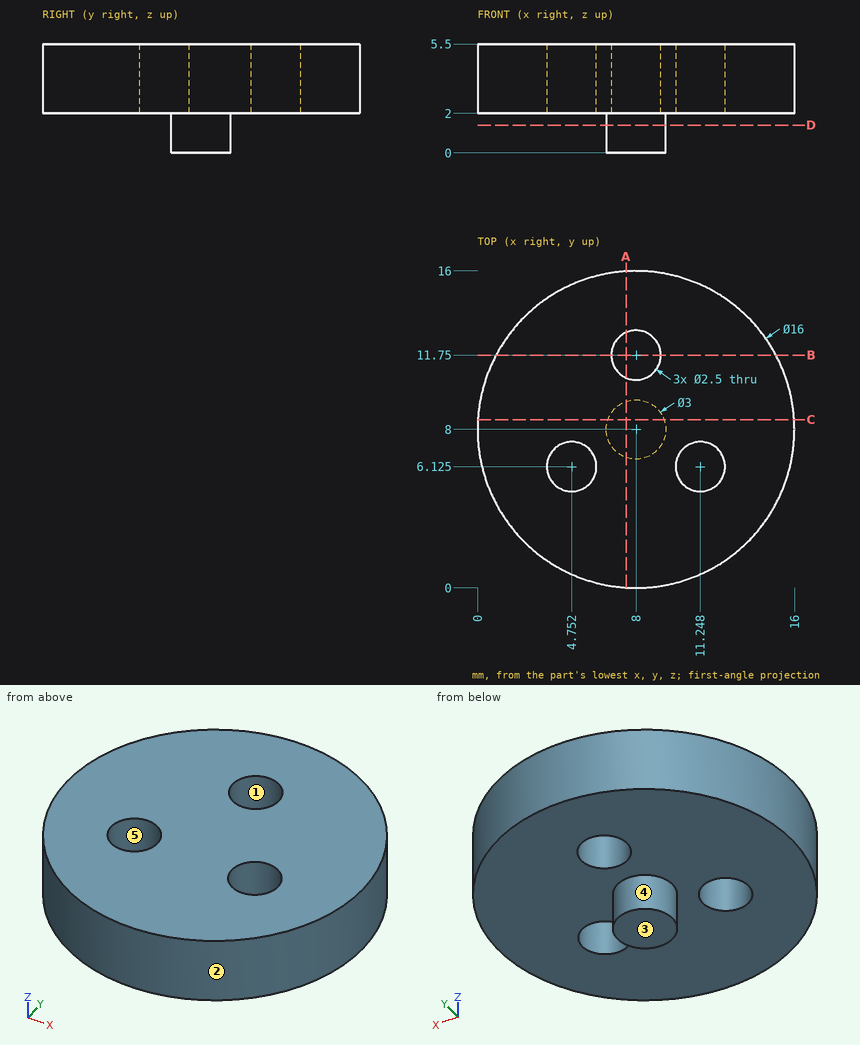
Geometry check sheet. Reference: drawing and pictorial views, mm from the part's lowest x, y, z. A direction names the side the tool comes from. Round coordinates to 2 decimals unless told otherwise and drop trailing zeros. Write each loop counter-clockwise with the first axis right and the second up, starting at its lowest first coordinate (ties: lowest second). Pieces come first, ordered by that corner, then holes.
Item 1: Section check B-B (y = 11.75). Record the boundary of the cut face in (x, z), plus the area to 3 significant figures.
Determined:
outline: (0.93, 2) - (6.75, 2) - (6.75, 5.5) - (0.93, 5.5) - close; (9.25, 2) - (15.07, 2) - (15.07, 5.5) - (9.25, 5.5) - close
area: 40.7 mm2
Item 2: Mould release check, pull along X, two halves, no side actions. Record for the marked faces 1, 2 and 3: +X half, -X half, draft (parallel to the pull), parting line (faces both ways), or undercut.
Determined:
face 1: undercut
face 2: parting line
face 3: draft
Item 3: Section check C-C (y = 8.5). Record the boundary of the cut face in (x, z) (1 decimal).
Determined:
outline: (0, 2) - (6.6, 2) - (6.6, 0) - (9.4, 0) - (9.4, 2) - (16, 2) - (16, 5.5) - (0, 5.5) - close
Item 4: Material ranges on line 1 along Z through (x, y) = (1.5, 10.5); line 2 along X through (y, z) = (5, 3.1) (1 decimal); line 3 along Y through (x, z) = (8.5, 2.4) (1 decimal), recorded low to high.
Determined:
line 1: z = 2 to 5.5
line 2: x = 0.6 to 4.2, 5.3 to 10.7, 11.8 to 15.4
line 3: y = 0 to 10.6, 12.9 to 16
Item 5: Go/stop test with flat-tipped pins: pin 1 Ø2 at (x, y) = (11.25, 6.12) entering from +Z; pin 2 Ø5 at (x, y) = (10, 4.5) entering from -Z; pin 3 Ø1 at (x, z) = (3.5, 3.5) entering from +Y; pin 4 Ø2 at (y, z) = (5.5, 2.5) entering from -X. Record where each tip stops, or that it passes through.
Determined:
pin 1: passes through
pin 2: stops at z = 2
pin 3: stops at y = 14.93
pin 4: stops at x = 0.14
Item 6: Access from +Z, -Z, +X, -X, +Y, -Y to the whole of each face (thin tool, end or side, straight path). Record for the marked faces 4 and 5.
Determined:
face 4: -Z
face 5: +Z, -Z
Item 7: Section check D-D (z = 1.4). Record the boundary of the cut face in (x, y).
Determined:
outline: circle Ø3 at (8, 8)
Item 8: Section check A-A (x = 7.5). Record the boundary of the cut face in (y, z) (1 decimal).
Determined:
outline: (0, 2) - (6.6, 2) - (6.6, 0) - (9.4, 0) - (9.4, 2) - (10.6, 2) - (10.6, 5.5) - (0, 5.5) - close; (12.9, 2) - (16, 2) - (16, 5.5) - (12.9, 5.5) - close
